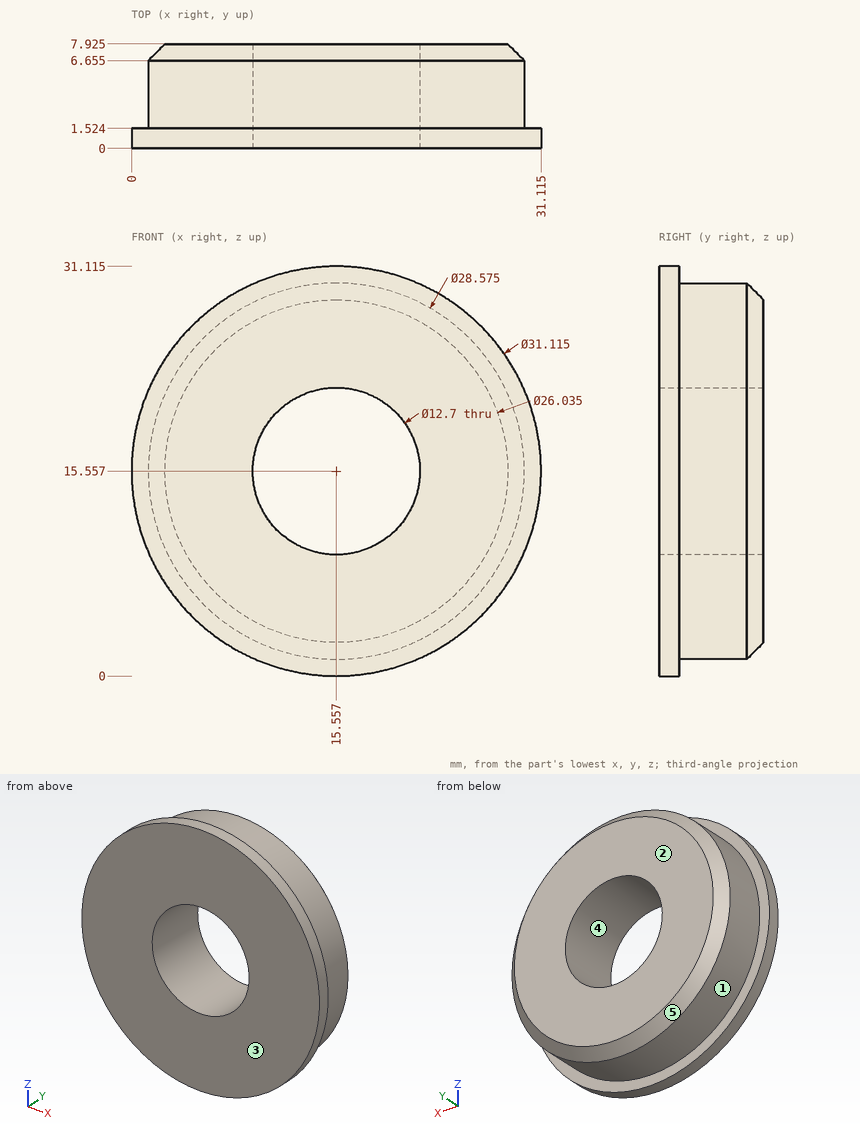
Verification items for this drawing (mm, ordinates from the low corner). A direction names the side the tool comes from. Give positions to 0.01 mm unless a question says otherwise; leave off trailing zeros. Answer as a JSON object with one key per item and string values. Group by question number.
1) Thickness scan on probe 1 along Z at (x, y) = (15.5, 1.25) (1 decimal); probe 2 along Y at (x, z) = (6, 4.5) (1 decimal); probe 3 along Z at (x, y) = (12.5, 3.25) (1 decimal). Record the ranges inside material, lowest first. Write a range as from..to.
2) Release check for a two-part mould opening along Z. For the marked faces 3, 4 and 5 record: pulls with the +Z half, pulls with the -Z half, needs draft (parallel to the pull), parting line crosses it, or undercut.
3) Depth check by flat-ended pin: P1, Ø9.5, axis at x = 10, z = 16.5, coming from the +Y side (1 decimal); P2, Ø1.5, axis at x = 13.5, y = 6, coming from the +Z side (1 decimal). Enter the tip coordinate at first touch or a pass-through.
4) Access from +Z, -Z, +X, -X, +Y, -Y to the whole of each face (thin tool, end or side, straight path). Record for the marked faces 1 and 2.
Geometry results:
{
 "1": {"probe 1": "z = 0..9.2, 21.9..31.1", "probe 2": "y = 0..1.5", "probe 3": "z = 1.6..10, 21.1..29.5"},
 "2": {"face 3": "needs draft", "face 4": "undercut", "face 5": "parting line crosses it"},
 "3": {"P1": "stops at y = 7.9", "P2": "stops at z = 29.8"},
 "4": {"face 1": "+Y", "face 2": "+Z, -Z, +X, -X, +Y"}
}
